Could you check a few things on this model? Use its own coordinates, in mm. Round coordinates to 2 decimals unless told otherwise and drop trailing zeros. Order: outer loops, then holes, each group sorted by start corner. A loop starts at its lowest first (then second) coordinate and runs counter-clockwise, first axis right, second up. Notation, with made-up numbers: M -16,47 L 32,47 A23 ccw 32,71 Z; hole C 60.25,-18.75 d5. An arc over 180 degrees is marked long. Write each question's results on one line, items separated by ' | '. Start each with the question number.
1. I'm going to push flat-ended pins straight in: pin 1 (1 mm diameter, centred on x = 37.5, y = 10.5, fed in from +Z); pin 2 (5 mm diameter, centred on x = 50, y = 4, fed in from +Z). Where does each tip first touch, or does it pass through?
2. Suppose I cut it at D-D on z = -12.5. Write out the boundary of the cut face in (x, y).
3. Suppose I cut it at A-A on y = 10.5. Write out the boundary of the cut face in (x, z) (3 decimals), and give its area (3 significant figures).
4. Please list where these lines run through material, in increasing order: L1, parallel to Z at x = -1.5, y = 1; L2, parallel to Z at x = 104, y = 12.25; L3, parallel to Z at x = 68, y = 3.
5. Suppose I cut it at C-C on x = 104.6. Write out the boundary of the cut face in (y, z), and give its area (3 significant figures).
6. Suppose I cut it at B-B on x = 4.6. Write out the boundary of the cut face in (y, z), and give its area (3 significant figures).
from build123d import *

# Parameters (mm, degrees)
BOSS_EXTRUDE1_DEPTH         = 12.7
F_1_4_20_TAPPED_HOLE1_D     = 5.1054
F_1_4_20_TAPPED_HOLE1_DEPTH = 19.05
F_1_4_20_TAPPED_HOLE1_TIP   = 1.533816902


with BuildPart() as part:
    # Sketch1 → Boss-Extrude1 (new body)
    with BuildSketch(Plane(origin=(0, 0, 0), x_dir=(1, 0, 0), z_dir=(0, 1, 0))):
        with BuildLine():
            Line((8.6875712, -23.868098094), (130.234472266, 20.372852858))
            ThreePointArc((130.234472266, 20.372852858), (155.303115466, 56.175), (130.234472266, 91.977147142))
            Line((130.234472266, 91.977147142), (8.6875712, 136.218098094))
            ThreePointArc((8.6875712, 136.218098094), (-14.568728351, 133.156541141), (-25.4, 112.35))
            Line((-25.4, 112.35), (-25.4, 0))
            ThreePointArc((-25.4, 0), (-14.568728351, -20.806541141), (8.6875712, -23.868098094))
        make_face()
    extrude(amount=BOSS_EXTRUDE1_DEPTH)

    # 1/4-20 Tapped Hole1
    with Locations(Plane(origin=(4.6, 12.7, -56.175), x_dir=(0, 0, 1), z_dir=(0, 1, 0))):
        with Locations((0, 0), (0, 100)):
            Hole(F_1_4_20_TAPPED_HOLE1_D / 2, depth=F_1_4_20_TAPPED_HOLE1_DEPTH)
            with Locations((0, 0, -(F_1_4_20_TAPPED_HOLE1_DEPTH + F_1_4_20_TAPPED_HOLE1_TIP / 2))):  # 118° drill point
                Cone(0, F_1_4_20_TAPPED_HOLE1_D / 2, F_1_4_20_TAPPED_HOLE1_TIP, mode=Mode.SUBTRACT)


solid = part.part
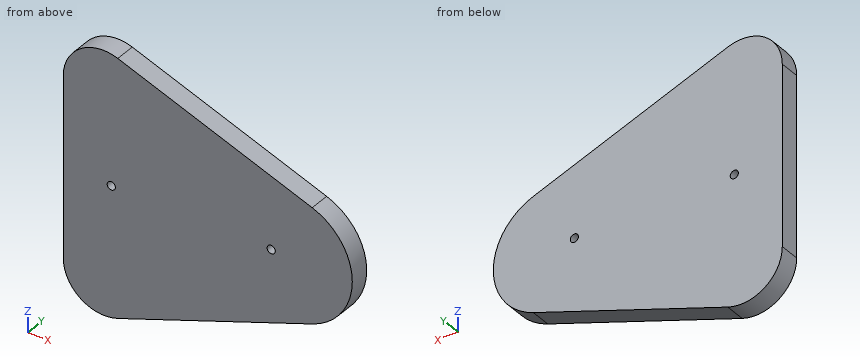
Filled sheet:
1) pin 1: stops at z = 13.56 | pin 2: stops at z = 9.74
2) outline: M -25.4,0 L 108.6,0 L 108.6,12.7 L -25.4,12.7 Z
3) outline: M -25.4,-112.35 A25.4 ccw 8.688,-136.218 L 130.234,-91.977 A38.1 ccw 130.234,-20.373 L 8.688,23.868 A25.4 ccw -25.4,0 Z; hole C 4.6,-56.175 d5.105; hole C 104.6,-56.175 d5.105 | area: 20,600 mm^2
4) L1: z = -137.71 to 25.36 | L2: z = -101.53 to -58.66, -53.69 to -10.82 | L3: z = -114.63 to 2.28
5) outline: M 0,-101.31 L 12.7,-101.31 L 12.7,-58.73 L 0,-58.73 Z; M 0,-53.62 L 12.7,-53.62 L 12.7,-11.04 L 0,-11.04 Z | area: 1,080 mm^2
6) outline: M 0,-137.33 L 12.7,-137.33 L 12.7,-58.73 L 0,-58.73 Z; M 0,-53.62 L 12.7,-53.62 L 12.7,24.98 L 0,24.98 Z | area: 2,000 mm^2
